Verification items for the finished model (mm, model axes). Face numbers are marked on the shaded views. A direction names the side the tool comes from. Coordinates: 2 decimals unless noted, no trailing zeros. Answer as a JSON object with one key per item and string values. Group by question number.
Q1. Cross-section at A-A on z = 38. Give the number of separate pieces and of enclosed holes in the cut face, and give its area (3 significant figures).
Q2. Set-up check for the marked faces 1, 2, 3 and 4: record each of +Z, -Z, +X, -X, +Y, -Y from which the full face is reachable in a straight line by a thin tool's end or side.
Q3. Gauge pin test, flat ends, axial feed: pin 1 Ø1.5 at (x, y) = (11, 20) entering from -Z; pin 2 Ø16 at (x, y) = (47.5, 39) entering from +Z; pin 3 Ø4 at (x, y) = (45.5, 20.5) entering from -Z; pin 4 Ø24 at (x, z) = (42.5, 37.5) entering from +Y. Record the tip position at first contact, or that the pin passes through.
Q4. Scan lines: L1, parallel to Y at x = 31.5, z = 29; L2, parallel to Y at x = 17, z = 26; L3, parallel to X at y = 4.5, z = 33. Record each from-to range of solid material in increasing order.
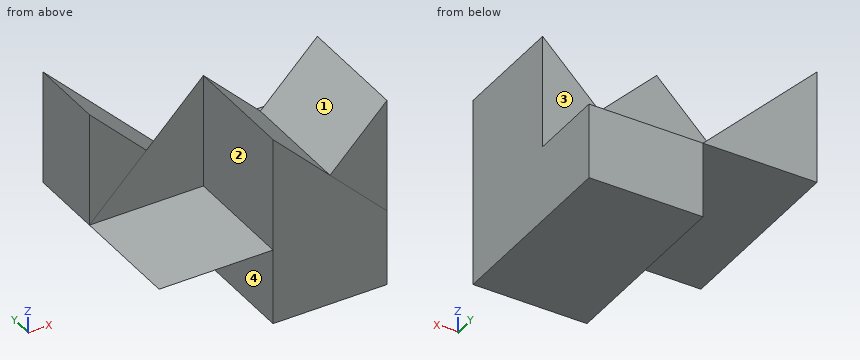
```python
from build123d import *

# Parameters (mm, degrees)
SKETCH1_W            = 60
SKETCH1_H            = 50
BOSS_EXTRUDE1_DEPTH  = 50
SKETCH2_W            = 30
SKETCH2_H            = 20
CUT_EXTRUDE1_DEPTH   = 50
CUT_EXTRUDE2_DEPTH   = 50
SKETCH5_W            = 30
SKETCH5_H            = 20
CUT_EXTRUDE6_DEPTH   = 29.999
SKETCH7_W            = 29.999
SKETCH7_H            = 29.999
CUT_EXTRUDE10_DEPTH  = 29.999
CUT_EXTRUDE11_DEPTH  = 20
BOSS_EXTRUDE5_DEPTH  = 20
CUT_EXTRUDE17_DEPTH  = 0.0001
CUT_EXTRUDE18_DEPTH  = 0.0001
BOSS_EXTRUDE16_DEPTH = 0.0001


with BuildPart() as part:
    # Sketch1 → Boss-Extrude1 (new body)
    with BuildSketch(Plane.XY):
        with Locations((30, 25)):
            Rectangle(SKETCH1_W, SKETCH1_H)
    extrude(amount=BOSS_EXTRUDE1_DEPTH)

    # Sketch2 → Cut-Extrude1 (cut)
    with BuildSketch(Plane(origin=(0, 50, 0), x_dir=(1, 0, 0), z_dir=(0, 1, 0))):
        with Locations((15, -10)):
            Rectangle(SKETCH2_W, SKETCH2_H)
    extrude(amount=-CUT_EXTRUDE1_DEPTH, mode=Mode.SUBTRACT)

    # Sketch3 → Cut-Extrude2 (cut)
    with BuildSketch(Plane(origin=(0, 50, 0), x_dir=(1, 0, 0), z_dir=(0, 1, 0))):
        Polygon((15, -35), (0, -50), (30, -50), align=None)
        Polygon((45, -35), (30, -50), (60, -50), align=None)
    extrude(amount=-CUT_EXTRUDE2_DEPTH, mode=Mode.SUBTRACT)

    # Sketch5 → Cut-Extrude6 (cut)
    with BuildSketch(Plane.XY.offset(50)):
        with Locations((45, 40)):
            Rectangle(SKETCH5_W, SKETCH5_H)
    extrude(amount=-CUT_EXTRUDE6_DEPTH, mode=Mode.SUBTRACT)

    # Sketch7 → Cut-Extrude10 (cut)
    with BuildSketch(Plane.XY.offset(50)):
        with Locations((14.9995, 14.9995)):
            Rectangle(SKETCH7_W, SKETCH7_H)
    extrude(amount=-CUT_EXTRUDE10_DEPTH, mode=Mode.SUBTRACT)

    # Sketch8 → Cut-Extrude11 (cut)
    with BuildSketch(Plane(origin=(0, 50, 0), x_dir=(1, 0, 0), z_dir=(0, 1, 0))):
        Polygon((15, -35), (30, -20.001), (44.999, -35.001), (30, -50), align=None)
    extrude(amount=-CUT_EXTRUDE11_DEPTH, mode=Mode.SUBTRACT)

    # Sketch11 → Boss-Extrude5 (add)
    with BuildSketch(Plane(origin=(0, 50, 0), x_dir=(1, 0, 0), z_dir=(0, 1, 0))):
        Polygon((0, -50), (0, -20), (30, -20.001), align=None)
    extrude(amount=-BOSS_EXTRUDE5_DEPTH)

    # Sketch14 → Cut-Extrude17 (cut)
    with BuildSketch(Plane(origin=(0, 29.999, 0), x_dir=(-1, 0, 0), z_dir=(0, -1, 0))):
        Polygon((-15, -35), (0, -20.001), (0, -50), align=None)
    extrude(amount=-CUT_EXTRUDE17_DEPTH, mode=Mode.SUBTRACT)

    # Sketch15 → Cut-Extrude18 (cut)
    with BuildSketch(Plane(origin=(0, 0, 0), x_dir=(-1, 0, 0), z_dir=(0, -1, 0))):
        Polygon((-45, -35), (-60, -20), (-60, -50), align=None)
    extrude(amount=-CUT_EXTRUDE18_DEPTH, mode=Mode.SUBTRACT)

    # Sketch16 → Boss-Extrude16 (add)
    with BuildSketch(Plane(origin=(0, 30, 0), x_dir=(1, 0, 0), z_dir=(0, 1, 0))):
        Polygon((45, -35), (30, -20.001), (15.000250004, -35.000250004), (30, -50), align=None)
    extrude(amount=BOSS_EXTRUDE16_DEPTH)


solid = part.part
```
Computed values:
{
 "1": {"separate pieces": "3", "enclosed holes": "0", "area": "960 mm²"},
 "2": {"face 1": "+Z, +Y, -Y", "face 2": "+Z, -X, -Y", "face 3": "+Z, +X, +Y", "face 4": "-Z, -X, +Y, -Y"},
 "3": {"pin 1": "stops at z = 20", "pin 2": "stops at z = 20", "pin 3": "stops at z = 0", "pin 4": "stops at y = 30"},
 "4": {"L1": "y = 0 to 30", "L2": "y = 30 to 50", "L3": "x = 30 to 60"}
}
